Check sheet for the modelled part. Datum: model origin and axes. Units: mm. Face numbers are marked on the shaded views. Round coordinates to 2 decimals unless told otherwise and drop trailing zeros. Write each loop counter-clockwise with the first axis right and the second up, starting at its lowest first coordinate (ties: lowest second). Pieces come first, ordered by that corner, then holes. Notation, with made-up numbers: (-4, 72) -> (1, 72) arc R14 cw to (1, 78) -> close; hole circle Ø4 at (-27.75, 88.5). An arc over 180 degrees is marked (long way). One line per item, written item: value.
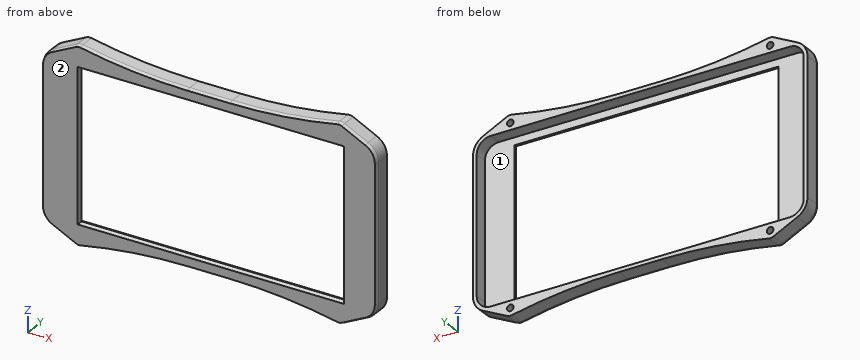
from build123d import *

# Parameters (mm, degrees)
EXTRUDE_1_DEPTH       = 2
EXTRUDE_2_DEPTH       = 8
SKETCH_6_R            = 3.5
SKETCH_6_R_2          = 1.5
EXTRUDE_10_DEPTH      = 8
SKETCH_7_W            = 121.7
SKETCH_7_H            = 68.8
CUT_EXTRUDE_1_DEPTH   = 10
FILLET_1_R            = 250
SKETCH_6_2_R          = 1.5
EXTRUDE_11_DEPTH      = 1.5
CHAMFER_1_SIZE        = 0.6
CHAMFER_1_SIZE2       = 1.648486452
CUT_EXTRUDE_START     = -6
CUT_EXTRUDE_1_2_DEPTH = 6


with BuildPart() as part:
    # 草图1 → 凸台-拉伸1 (new body)
    with BuildSketch(Plane(origin=(0, 0, 0), x_dir=(1, 0, 0), z_dir=(0, 1, 0))):
        with BuildLine():
            Line((6, 0.2), (143.8, 0.2))
            ThreePointArc((143.8, 0.2), (148.184062043, -1.615937957), (150, -6))
            Line((150, -6), (150, -68.8))
            ThreePointArc((150, -68.8), (148.184062043, -73.184062043), (143.8, -75))
            Line((143.8, -75), (6, -75))
            ThreePointArc((6, -75), (1.615937957, -73.184062043), (-0.2, -68.8))
            Line((-0.2, -68.8), (-0.2, -6))
            ThreePointArc((-0.2, -6), (1.615937957, -1.615937957), (6, 0.2))
        make_face()
    extrude(amount=EXTRUDE_1_DEPTH)

    # 草图1<5> → 拉伸-薄壁2 (add)
    with BuildSketch(Plane(origin=(0, 0, 0), x_dir=(1, 0, 0), z_dir=(0, 1, 0))):
        with BuildLine():
            Line((6, 2.2), (143.8, 2.2))
            ThreePointArc((143.8, 2.2), (149.598275606, -0.201724394), (152, -6))
            Line((152, -6), (152, -68.8))
            ThreePointArc((152, -68.8), (149.598275606, -74.598275606), (143.8, -77))
            Line((143.8, -77), (6, -77))
            ThreePointArc((6, -77), (0.201724394, -74.598275606), (-2.2, -68.8))
            Line((-2.2, -68.8), (-2.2, -6))
            ThreePointArc((-2.2, -6), (0.201724394, -0.201724394), (6, 2.2))
        make_face()
        with BuildLine():
            Line((6, 0.2), (143.8, 0.2))
            ThreePointArc((143.8, 0.2), (148.184062043, -1.615937957), (150, -6))
            Line((150, -6), (150, -68.8))
            ThreePointArc((150, -68.8), (148.184062043, -73.184062043), (143.8, -75))
            Line((143.8, -75), (6, -75))
            ThreePointArc((6, -75), (1.615937957, -73.184062043), (-0.2, -68.8))
            Line((-0.2, -68.8), (-0.2, -6))
            ThreePointArc((-0.2, -6), (1.615937957, -1.615937957), (6, 0.2))
        make_face(mode=Mode.SUBTRACT)
    extrude(amount=EXTRUDE_2_DEPTH)

    # 草图6 → 凸台-拉伸10 (add)
    # profile 1 of 4: a face of its own
    with BuildSketch(Plane(origin=(0, 0, 0), x_dir=(1, 0, 0), z_dir=(0, 1, 0))):
        with Locations((15, 3.7)):
            Circle(SKETCH_6_R)
        with Locations(Location((15, 3.7, 0), (0, 0, 90))):
            Circle(SKETCH_6_R_2, mode=Mode.SUBTRACT)
    # profile 2 of 4: a face of its own
    with BuildSketch(Plane(origin=(0, 0, 0), x_dir=(1, 0, 0), z_dir=(0, 1, 0))):
        with Locations((15, -78.5)):
            Circle(SKETCH_6_R)
        with Locations(Location((15, -78.5, 0), (0, 0, 90))):
            Circle(SKETCH_6_R_2, mode=Mode.SUBTRACT)
    # profile 3 of 4: a face of its own
    with BuildSketch(Plane(origin=(0, 0, 0), x_dir=(1, 0, 0), z_dir=(0, 1, 0))):
        with Locations((134.8, 3.7)):
            Circle(SKETCH_6_R)
        with Locations(Location((134.8, 3.7, 0), (0, 0, 90))):
            Circle(SKETCH_6_R_2, mode=Mode.SUBTRACT)
    # profile 4 of 4: a face of its own
    with BuildSketch(Plane(origin=(0, 0, 0), x_dir=(1, 0, 0), z_dir=(0, 1, 0))):
        with Locations((134.8, -78.5)):
            Circle(SKETCH_6_R)
        with Locations(Location((134.8, -78.5, 0), (0, 0, 90))):
            Circle(SKETCH_6_R_2, mode=Mode.SUBTRACT)
    extrude(amount=EXTRUDE_10_DEPTH)

    # 草图7 → Cut-Extrude 1 (cut)
    with BuildSketch(Plane(origin=(0, 0, 0), x_dir=(-1, 0, 0), z_dir=(0, -1, 0))):
        with Locations((-75.85, -37.4)):
            Rectangle(SKETCH_7_W, SKETCH_7_H)
    extrude(amount=-CUT_EXTRUDE_1_DEPTH, mode=Mode.SUBTRACT)

    # 圆角1
    fillet_1_edges = [part.edges().sort_by_distance(p)[0] for p in [
        (18.16227766, 4, 77),
        (11.83772234, 4, 77),
        (137.96227766, 4, 77),
        (131.63772234, 4, 77),
        (131.63772234, 4, -2.2),
        (137.96227766, 4, -2.2),
        (11.83772234, 4, -2.2),
        (18.16227766, 4, -2.2),
    ]]
    fillet(fillet_1_edges, radius=FILLET_1_R)

    # 草图6<2> → 凸台-拉伸11 (add)
    with BuildSketch(Plane(origin=(0, 0, 0), x_dir=(1, 0, 0), z_dir=(0, 1, 0))):
        with Locations(Location((15, 3.7, 0), (0, 0, 90))):
            Circle(SKETCH_6_2_R)
        with Locations(Location((15, -78.5, 0), (0, 0, 90))):
            Circle(SKETCH_6_2_R)
        with Locations(Location((134.8, 3.7, 0), (0, 0, 90))):
            Circle(SKETCH_6_2_R)
        with Locations(Location((134.8, -78.5, 0), (0, 0, 90))):
            Circle(SKETCH_6_2_R)
    extrude(amount=EXTRUDE_11_DEPTH)

    # 倒角1
    chamfer_1_edges = [part.edges().sort_by_distance(p)[0] for p in [
        (136.7, 0, 37.4),
        (75.85, 0, 71.8),
        (15, 0, 37.4),
        (75.85, 0, 3),
        (14.502874151, 0, 81.964515246),
        (74.9, 0, 77),
        (135.297125849, 0, 81.964515246),
        (150.714252509, 0, 73.20830038),
        (135.297125849, 0, -7.164515246),
        (74.9, 0, -2.2),
        (14.502874151, 0, -7.164515246),
        (-0.914252509, 0, 1.59169962),
        (7.988030543, 0, 78.850628869),
        (40.273083878, 0, 78.235796001),
        (141.811969457, 0, 78.850628869),
        (109.526916122, 0, 78.235796001),
        (141.811969457, 0, -4.050628869),
        (109.526916122, 0, -3.435796001),
        (7.988030543, 0, -4.050628869),
        (40.273083878, 0, -3.435796001),
        (-2.2, 0, 37.4),
        (-0.914252509, 0, 73.20830038),
        (152, 0, 37.4),
        (150.714252509, 0, 1.59169962),
    ]]
    chamfer_1_side = [part.faces().sort_by_distance(p)[0] for p in [
        (0.58783664, 0, 72.250617658),
    ]]
    chamfer(chamfer_1_edges, length=CHAMFER_1_SIZE, length2=CHAMFER_1_SIZE2, reference=chamfer_1_side[0])

    # 草图11 → Cut-Extrude 1 2 (cut)
    with BuildSketch(Plane(origin=(0, 8, 0), x_dir=(1, 0, 0), z_dir=(0, 1, 0)).offset(CUT_EXTRUDE_START)):
        with BuildLine():
            Line((143.8, 0.5), (6, 0.5))
            ThreePointArc((6, 0.5), (1.403805922, -1.403805922), (-0.5, -6))
            Line((-0.5, -6), (-0.5, -68.8))
            ThreePointArc((-0.5, -68.8), (1.403805922, -73.396194078), (6, -75.3))
            Line((6, -75.3), (143.8, -75.3))
            ThreePointArc((143.8, -75.3), (148.396194078, -73.396194078), (150.3, -68.8))
            Line((150.3, -68.8), (150.3, -6))
            ThreePointArc((150.3, -6), (148.396194078, -1.403805922), (143.8, 0.5))
        make_face()
        with BuildLine():
            Line((143.8, 0.2), (6, 0.2))
            ThreePointArc((6, 0.2), (1.615937957, -1.615937957), (-0.2, -6))
            Line((-0.2, -6), (-0.2, -68.8))
            ThreePointArc((-0.2, -68.8), (1.615937957, -73.184062043), (6, -75))
            Line((6, -75), (143.8, -75))
            ThreePointArc((143.8, -75), (148.184062043, -73.184062043), (150, -68.8))
            Line((150, -68.8), (150, -6))
            ThreePointArc((150, -6), (148.184062043, -1.615937957), (143.8, 0.2))
        make_face(mode=Mode.SUBTRACT)
    extrude(amount=CUT_EXTRUDE_1_2_DEPTH, mode=Mode.SUBTRACT)


solid = part.part
Item 1: Sectioned sample at C-C on y = 6.5. Count the separate pieces of the cut face and the enclosed holes in it, and give its area (3 significant figures).
Answer:
separate pieces: 1
enclosed holes: 5
area: 1,190 mm^2
Item 2: Mould release check, pull along X, two halves, no side actions. Record for the marked faces 1 and 2: pulls with the +X half, pulls with the -X half, needs draft (parallel to the pull), parting line crosses it, or undercut.
Answer:
face 1: undercut
face 2: needs draft
Item 3: Sectioned sample at A-A on z = 34.5. Enter the section's corners in (x, y), and give its area (3 significant figures).
Answer:
outline: (-2.2, 1.65) -> (-1.6, 0) -> (14.4, 0) -> (15, 1.65) -> (15, 2) -> (-0.5, 2) -> (-0.5, 8) -> (-2.2, 8) -> close; (136.7, 1.65) -> (137.3, 0) -> (151.4, 0) -> (152, 1.65) -> (152, 8) -> (150.3, 8) -> (150.3, 2) -> (136.7, 2) -> close
area: 83.4 mm^2
Item 4: Depth check by flat-ended pin: P1, Ø3, axis at x = 108, y = 4, coming from the +Z side; P2, Ø1.9, axis at x = 74, y = 4.5, coming from the +Z side; P3, Ø3, axis at x = 19, z = 71, coming from the +Y side. Enter the tip coordinate at first touch or a pass-through.
Answer:
P1: stops at z = 78.23
P2: stops at z = 77
P3: stops at y = 2
Item 5: Thickness scan on line 1 (Z direction, x = 15, y = 3.5); line 2 (X direction, y = 3, z = 42); line 3 (Y direction, x = 138, z = 41). Record the ranges inside material, lowest first.
Answer:
line 1: z = -7.2 to -5.2, -2.2 to -0.5, 75.3 to 77, 80 to 82
line 2: x = -2.2 to -0.5, 150.3 to 152
line 3: y = 0 to 2
Item 6: Sectioned sample at B-B on x = 78. Enter the section's corners in (y, z), and give its area (3 significant figures).
Answer:
outline: (0, -1.6) -> (1.65, -2.2) -> (8, -2.2) -> (8, -0.5) -> (2, -0.5) -> (2, 3) -> (1.65, 3) -> (0, 2.4) -> close; (0, 72.4) -> (1.65, 71.8) -> (2, 71.8) -> (2, 75.3) -> (8, 75.3) -> (8, 77) -> (1.65, 77) -> (0, 76.4) -> close
area: 39.2 mm^2
